Check sheet for the modelled part. Datum: model origin and axes. Units: mm. Round coordinates to 2 decimals unless told otherwise and drop trailing zeros. Loops run counter-clockwise (first coordinate to the right, second up) from the corner with the lowest first, then second, coordinate; pieces in that order, holes last. Notation, with made-up numbers: (8.25, 7) - (44.25, 7) arc R32 cw to (44.25, 37) - close; hole circle Ø2 at (-36.75, 43). An arc over 180 degrees is marked (long way). Put each result on its own line as item: value. Start each with the question number.
Item 1: Gauge pin test, flat ends, axial feed: pin 1 Ø2 at (x, y) = (90.5, 1) entering from -Z; pin 2 Ø2 at (y, z) = (2, 21) entering from +X; pin 3 Ø1.5 at (y, z) = (0.5, 8.5) entering from +X. Record the tip position at first contact, or that the pin passes through.
Item 2: Material ranges on line 1 along X through (y, z) = (2.55, 2.5); line 2 along X through (y, z) = (2.8, 9.5); line 3 along Z through (x, y) = (91, 3.4), recorded low to high.
Item 3: Section check B-B, the plane y = 0.6. Record the cut outline in (x, z).
Item 4: Section check D-D, the plane z = 17. Record the cut outline in (x, y).
Item 5: Section check A-A, the plane z = 5. Record the cut outline in (x, y).
Item 6: Section check C-C, the plane x = 229.5. Record the cut outline in (y, z).
Autodesk Fusion 360 part; units mm, degrees
sketch "Sketch1" plane through (0, 0, 0) normal (0, 1, 0) x (1, 0, 0)
  line L0 (0, 0) -> (0, -50)
  line L1 (0, -50) -> (300, -50)
  line L2 (0, 0) -> (50, 0)
  line L3 (50, 0) -> (50, -30)
  line L4 (50, -30) -> (125, -30)
  line L5 (125, -30) -> (125, 0)
  line L6 (125, 0) -> (160, 0)
  line L7 (160, 0) -> (160, -30)
  line L8 (160, -30) -> (235, -30)
  line L9 (235, -30) -> (235, 0)
  line L10 (235, 0) -> (281.5957, 0)
  line L11 (299.4269, -50.5394) -> (300, -50)
  line L12 (0, 0) -> (350, 0) construction
  line L13 (281.5957, 0) -> (310, -30) construction
  line L14 (310, -30) -> (300, -50) construction
  line L15 (281.5957, 0) -> (310, -30)
  line L16 (300, -50) -> (310, -30)
  dimension "d1" = 50
  dimension "d2" = 300
  dimension "d3" = 50
  dimension "d4" = 30
  dimension "d5" = 75
  dimension "d6" = 35
  dimension "d7" = 75
  dimension "d11" = 30
  dimension "d12" = 30
  dimension "d13" = 350
  dimension "d16" = 30
  dimension "d17" = 30
  dimension "d19" = 110
  dimension "d20" = 41.3135
extrude "Extrude1" add sketch "Sketch1" along normal blind 4
Check result:
1. pin 1: z = 30
1. pin 2: x = 302.43
1. pin 3: x = 290.35
2. line 1: 0 to 50, 125 to 160, 235 to 283.96
2. line 2: 0 to 50, 125 to 160, 235 to 290.59
2. line 3: 30 to 50
3. outline: (0, 0) - (50, 0) - (50, 30) - (125, 30) - (125, 0) - (160, 0) - (160, 30) - (235, 30) - (235, 0) - (281.6, 0) - (310, 30) - (300, 50) - (0, 50) - close
4. outline: (0, 0) - (50, 0) - (50, 4) - (0, 4) - close; (125, 0) - (160, 0) - (160, 4) - (125, 4) - close; (235, 0) - (297.69, 0) - (297.69, 4) - (235, 4) - close
5. outline: (0, 0) - (50, 0) - (50, 4) - (0, 4) - close; (125, 0) - (160, 0) - (160, 4) - (125, 4) - close; (235, 0) - (286.33, 0) - (286.33, 4) - (235, 4) - close
6. outline: (0, 30) - (4, 30) - (4, 50) - (0, 50) - close
